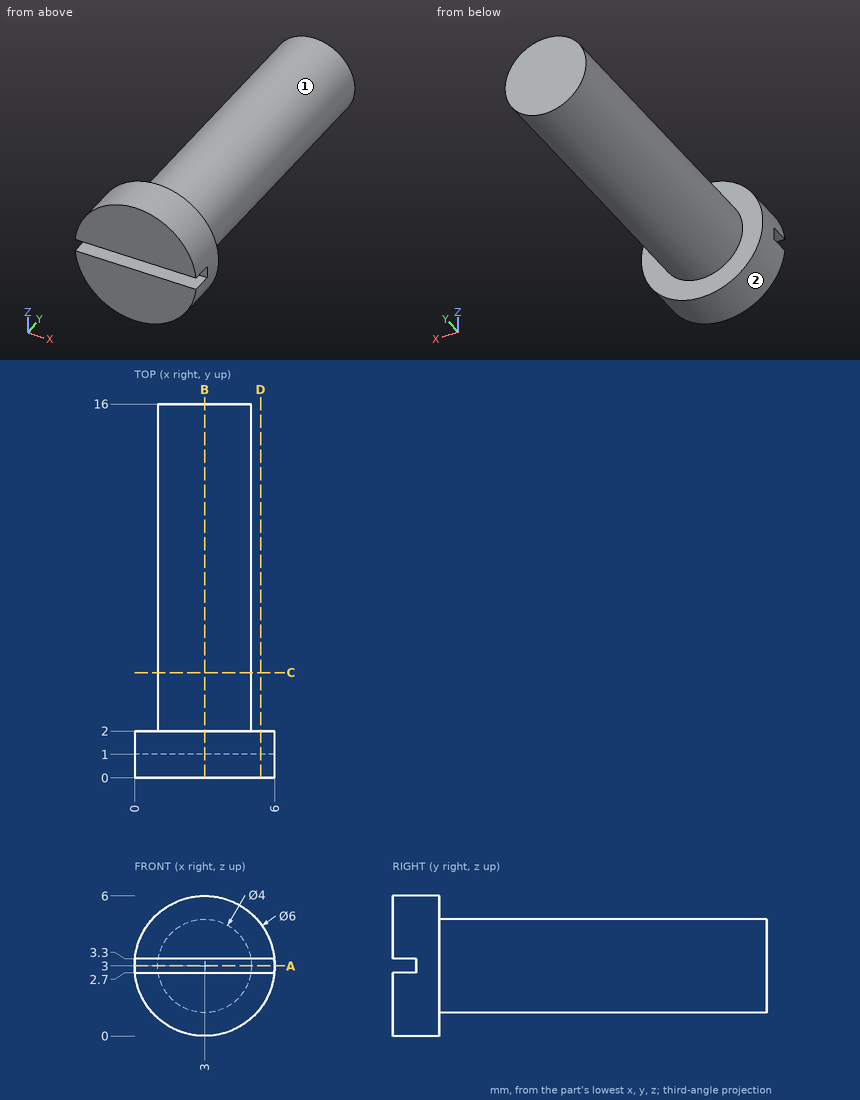
Answer from the drawing. Dimensions are ordinates in mm from the lowest x, y and z of the part. A direction names the side the tool comes from. Give positions to 0.01 mm unless a question says otherwise; leave off trailing zeros. Loops run counter-clockwise (first coordinate to the right, second up) from the corner with the lowest first, then second, coordinate; pieces in that order, holes last. Notation, with made-up numbers: (-27, 80) -> (-9, 80) arc R5 cw to (-9, 86) -> close; hole circle Ø3 at (79, 29.5). An arc over 180 degrees is marked (long way). One line per question, with ' | ' between items. Start each with the question number.
1) Section B-B, the plane x = 3 is taken. Determine the outline of the cut face in (y, z), then the cut area to 3 significant figures.
2) For the marked faces 1 and 2, determine the directions among +Z, -Z, +X, -X, +Y, -Y from which every point of the face is accessible in a straight line to the end or side of a thin tool.
3) Each of these flat-tipped pins is pushed along its axis until it touches: pin 1 (0.5 mm diameter, centred on x = 2.5, y = 0.5, fed in from -Z); pin 2 (1.5 mm diameter, centred on y = 3, z = 2, fed in from -X). Where does it stop, or does it pass through?
4) Section A-A, the plane z = 3 is taken. Determine the outline of the cut face in (x, y).
5) Section C-C, the plane y = 4.5 is taken. Determine the outline of the cut face in (x, z).
6) Section D-D, the plane x = 5.4 is taken. Determine the outline of the cut face in (y, z).
7) Straight lines are drawn through the part: L1, parallel to Y at x = 4.3, z = 5.3; L2, parallel to Y at x = 1.55, z = 3.2; L3, parallel to X at y = 5.75, z = 4.2. For each, find the intervals that lie inside material, in ascending order.
Resolved:
1) outline: (0, 0) -> (2, 0) -> (2, 1) -> (16, 1) -> (16, 5) -> (2, 5) -> (2, 6) -> (0, 6) -> (0, 3.3) -> (1, 3.3) -> (1, 2.7) -> (0, 2.7) -> close | area: 67.4 mm2
2) face 1: +Y | face 2: +Y, -Y
3) pin 1: z = 0.01 | pin 2: x = 1.02
4) outline: (0, 1) -> (6, 1) -> (6, 2) -> (5, 2) -> (5, 16) -> (1, 16) -> (1, 2) -> (0, 2) -> close
5) outline: circle Ø4 at (3, 3)
6) outline: (0, 1.2) -> (2, 1.2) -> (2, 4.8) -> (0, 4.8) -> (0, 3.3) -> (1, 3.3) -> (1, 2.7) -> (0, 2.7) -> close
7) L1: 0 to 2 | L2: 1 to 16 | L3: 1.4 to 4.6
